The model under review builds one solid part; all positions refer to its coordinate system, in mm. Face numbers are marked on the shaded views. A direction names the side the tool comes from. Round coordinates to 2 decimals unless told otherwise and drop trailing zeros. Write each loop counter-clockwise with the first axis right and the second up, starting at its lowest first coordinate (ties: lowest second). Pieces come first, ordered by that corner, then holes. Notation, with made-up numbers: M 37.5,-34 L 80.5,-34 A17 ccw 80.5,-21 Z; hole C 59.25,-22 d1. An arc over 180 degrees is marked long. One line per item, written item: value. Start each with the question number.
1) Tool access review of the marked faces 4, 5, 6 and 7: name each direction out of +Z, -Z, +X, -X, +Y, -Y from which nothing blocks a thin tool from reaching the whole face with its end or side.
2) Wall thickness on probe 1 along X at (y, z) = (10.5, -10); probe 2 along X at (y, z) = (0, 6.5); probe 3 along Y at (x, z) = (5.35, -8.35): over which ranges is each line inside the solid? List them lowest first.
3) Mouldability with a two-part tool opening along Z and no side actions: class the marked faces 1, 2 and 3 as +Z half, -Z half, draft (parallel to the pull), parting line (faces both ways), or undercut.
4) For P1, Ø0.9, axis at x = 3, z = -5, coming from the +Y side; P2, Ø16, axis at y = 13, z = -3.5, coming from the -X side; P3, Ø1.5, axis at x = 0.5, z = 5, coming from the -Y side; P4, Ø8, axis at x = 2, y = 9, coming from the +Z side, all flat-tipped, find the tip position at first contact; note any pin that passes through.
5) Take a section at C-C, the plane x = -0.75. Write out the cut boundary in (y, z).
6) Take a section at D-D, the plane z = -1.5. Write out the cut boundary in (x, y).
7) Take a section at B-B, the plane y = 5.5. Write out the cut boundary in (x, z).
8) Take a section at A-A, the plane z = 8.35. Write out the cut boundary in (x, y).
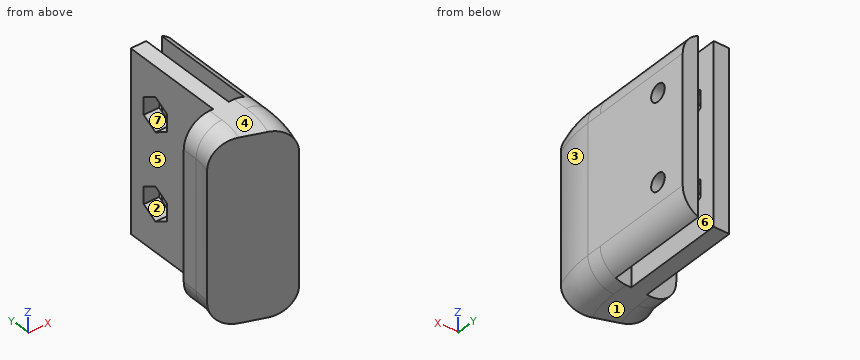
from build123d import *

# Parameters (mm, degrees)
BOSS_EXTRU_1_DEPTH      = 3
R_VOLUTION1_ANGLE       = 20
ESQUISSE5_W             = 3
ESQUISSE5_H             = 34.7
BOSS_EXTRU_2_DEPTH      = 20
ESQUISSE6_R             = 1.65
ENL_V_MAT_EXTRU_1_DEPTH = 16.303073792
ENL_V_MAT_EXTRU_3_REACH = 11


with BuildPart() as part:
    # Esquisse1 → Boss.-Extru.1 (new body)
    with BuildSketch(Plane(origin=(0, 0, 0), x_dir=(1, 0, 0), z_dir=(0, 1, 0))):
        with BuildLine():
            Line((2.35, -17.35), (-2.35, -17.35))
            ThreePointArc((-2.35, -17.35), (-5.885533906, -15.885533906), (-7.35, -12.35))
            Line((-7.35, -12.35), (-7.35, 12.35))
            ThreePointArc((-7.35, 12.35), (-5.885533906, 15.885533906), (-2.35, 17.35))
            Line((-2.35, 17.35), (2.35, 17.35))
            ThreePointArc((2.35, 17.35), (5.885533906, 15.885533906), (7.35, 12.35))
            Line((7.35, 12.35), (7.35, -12.35))
            ThreePointArc((7.35, -12.35), (5.885533906, -15.885533906), (2.35, -17.35))
        make_face()
    extrude(amount=BOSS_EXTRU_1_DEPTH)

    # Esquisse4 → Révolution1 (revolve)
    with BuildSketch(Plane.XZ):
        with BuildLine():
            Line((2.35, -17.35), (-2.35, -17.35))
            ThreePointArc((-2.35, -17.35), (-5.885533906, -15.885533906), (-7.35, -12.35))
            Line((-7.35, -12.35), (-7.35, 12.35))
            ThreePointArc((-7.35, 12.35), (-5.885533906, 15.885533906), (-2.35, 17.35))
            Line((-2.35, 17.35), (2.35, 17.35))
            ThreePointArc((2.35, 17.35), (5.885533906, 15.885533906), (7.35, 12.35))
            Line((7.35, 12.35), (7.35, -12.35))
            ThreePointArc((7.35, -12.35), (5.885533906, -15.885533906), (2.35, -17.35))
        make_face()
    revolve(axis=Axis((-17.35, 0, 12.35), (0, 0, -1)), revolution_arc=R_VOLUTION1_ANGLE)

    # Esquisse5 → Boss.-Extru.2 (add)
    with BuildSketch(Plane(origin=(0, 3, 0), x_dir=(1, 0, 0), z_dir=(0, 1, 0))):
        with Locations((-0.15, 0)):
            Rectangle(ESQUISSE5_W, ESQUISSE5_H)
        with BuildLine():
            Line((7.35, -12.35), (7.35, 12.35))
            ThreePointArc((7.35, 12.35), (6.533300133, 15.088612788), (4.35, 16.932575695))
            Line((4.35, 16.932575695), (4.35, -16.932575695))
            ThreePointArc((4.35, -16.932575695), (6.533300133, -15.088612788), (7.35, -12.35))
        make_face()
    extrude(amount=BOSS_EXTRU_2_DEPTH)

    # Esquisse6 → Enlèv. mat.-Extru.1 (cut, through all)
    with BuildSketch(Plane(origin=(7.35, 0, 0), x_dir=(0, 0, -1), z_dir=(1, 0, 0))):
        with Locations((-8.35, 17)):
            Circle(ESQUISSE6_R)
        with Locations((8.35, 17)):
            Circle(ESQUISSE6_R)
    extrude(amount=-ENL_V_MAT_EXTRU_1_DEPTH, mode=Mode.SUBTRACT)

    # Esquisse8 → Enlèv. mat.-Extru.3 (cut, up to next)
    with BuildSketch(Plane.ZY.offset(1.65), mode=Mode.PRIVATE) as enl_v_mat_extru_3_sk1:
        Polygon((-6.704551733, 19.85), (-9.995448267, 19.85), (-11.640896534, 17), (-9.995448267, 14.15), (-6.704551733, 14.15), (-5.059103466, 17), align=None)
    enl_v_mat_extru_3_tool1 = extrude(enl_v_mat_extru_3_sk1.sketch, amount=-ENL_V_MAT_EXTRU_3_REACH, mode=Mode.PRIVATE) & part.part
    add(enl_v_mat_extru_3_tool1.solids().sort_by_distance((-1.65, 17, -8.35))[0], mode=Mode.SUBTRACT)
    # Esquisse8 → Enlèv. mat.-Extru.3 (cut, up to next)
    with BuildSketch(Plane.ZY.offset(1.65), mode=Mode.PRIVATE) as enl_v_mat_extru_3_sk2:
        Polygon((9.995448267, 19.85), (6.704551733, 19.85), (5.059103466, 17), (6.704551733, 14.15), (9.995448267, 14.15), (11.640896534, 17), align=None)
    enl_v_mat_extru_3_tool2 = extrude(enl_v_mat_extru_3_sk2.sketch, amount=-ENL_V_MAT_EXTRU_3_REACH, mode=Mode.PRIVATE) & part.part
    add(enl_v_mat_extru_3_tool2.solids().sort_by_distance((-1.65, 17, 8.35))[0], mode=Mode.SUBTRACT)


solid = part.part
Checked values:
1. face 4: +Z, +X, -X, +Y, -Y
1. face 5: +Z, -Z, -X, +Y
1. face 6: +Z, -Z, +Y
1. face 7: -X
2. probe 1: x = -1.65 to 1.35, 4.35 to 7.35
2. probe 2: x = -7.35 to 7.35
2. probe 3: y = -8.26 to 15.35, 18.65 to 23
3. face 1: -Z half
3. face 2: undercut
3. face 3: draft
4. P1: stops at y = 3
4. P2: stops at x = -1.65
4. P3: stops at y = -6.77
4. P4: stops at z = 17.35
5. outline: M -6.04,-17.35 L 23,-17.35 L 23,17.35 L -6.04,17.35 Z; hole M 14.15,-10 L 17,-11.64 L 19.85,-10 L 19.85,-6.7 L 17,-5.06 L 14.15,-6.7 Z; hole M 14.15,6.7 L 17,5.06 L 19.85,6.7 L 19.85,10 L 17,11.64 L 14.15,10 Z
6. outline: M -7.95,-3.42 L 5.86,-8.45 A24.7 ccw 7.35,0 L 7.35,23 L 4.35,23 L 4.35,3 L 1.35,3 L 1.35,23 L -1.65,23 L -1.65,3 L -7.35,3 L -7.35,0 A10 cw Z
7. outline: M -1.65,-17.35 L 1.35,-17.35 L 1.35,17.35 L -1.65,17.35 Z; M 4.35,-16.93 A5 ccw 7.35,-12.35 L 7.35,12.35 A5 ccw 4.35,16.93 Z
8. outline: M -7.95,-3.42 L 5.86,-8.45 A24.7 ccw 7.35,0 L 7.35,15.35 L 4.35,15.35 L 4.35,3 L 1.35,3 L 1.35,14.15 L -1.65,14.15 L -1.65,3 L -7.35,3 L -7.35,0 A10 cw Z; M -1.65,19.85 L 1.35,19.85 L 1.35,23 L -1.65,23 Z; M 4.35,18.65 L 7.35,18.65 L 7.35,23 L 4.35,23 Z
